from build123d import *

# Parameters (mm, degrees)
BOSS_EXTRUDE1_DEPTH             = 50
SKETCH2_W                       = 109.146932236
SKETCH2_H                       = 60.735636093
CUT_EXTRUDE1_DEPTH              = 88.05
F_20_0_161_DIAMETER_HOLE1_D     = 4.0894
F_20_0_161_DIAMETER_HOLE1_DEPTH = 87.05
SKETCH7_W                       = 11
SKETCH7_H                       = 4
BOSS_EXTRUDE2_DEPTH             = 20
FILLET1_R                       = 2
SKETCH8_R                       = 5.5
BOSS_EXTRUDE3_DEPTH             = 8
BOSS_EXTRUDE3_DEPTH_BACK        = 12
FILLET2_R                       = 5


with BuildPart() as part:
    # Sketch1 → Boss-Extrude1 (new body)
    with BuildSketch(Plane.XY):
        with BuildLine():
            Line((-86.473709878, 10), (-83.956551263, 10))
            ThreePointArc((-83.956551263, 10), (-84.55, 0), (-83.956551263, -10))
            Line((-83.956551263, -10), (-86.473709878, -10))
            ThreePointArc((-86.473709878, -10), (-87.05, 0), (-86.473709878, 10))
        make_face()
    extrude(amount=BOSS_EXTRUDE1_DEPTH)

    # Sketch2 → Cut-Extrude1 (cut, through all)
    with BuildSketch(Plane(origin=(0, 0, 0), x_dir=(0, 0, -1), z_dir=(1, 0, 0))):
        with Locations((-34.220207601, -2.682367057)):
            Rectangle(SKETCH2_W, SKETCH2_H)
        Polygon((0, 10), (0, -10), (-5, -10), (-50, -2.5), (-50, 2.5), (-5, 10), align=None, mode=Mode.SUBTRACT)
    extrude(amount=-CUT_EXTRUDE1_DEPTH, mode=Mode.SUBTRACT)

    # #20 (0.161) Diameter Hole1
    with Locations(Plane(origin=(0, 0, 0), x_dir=(0, 0, -1), z_dir=(1, 0, 0))):
        with Locations((-46, 0), (-5, 6), (-5, -6), (-17.5, 0)):
            Hole(F_20_0_161_DIAMETER_HOLE1_D / 2, depth=F_20_0_161_DIAMETER_HOLE1_DEPTH)

    # Sketch7 → Boss-Extrude2 (add)
    with BuildSketch(Plane(origin=(-80, 0, -87.99983), x_dir=(0, 0, -1), z_dir=(1, 0, 0))):
        with Locations((-120.49983, 0)):
            Rectangle(SKETCH7_W, SKETCH7_H)
    extrude(amount=-BOSS_EXTRUDE2_DEPTH)

    # Fillet1
    fillet1_edges = [part.edges().sort_by_distance(p)[0] for p in [
        (-87.027021666, -2, 32.5),
        (-87.05, 0, 27),
        (-87.027021666, 2, 32.5),
        (-87.05, 0, 38),
    ]]
    fillet(fillet1_edges, radius=FILLET1_R)

    # Sketch8 → Boss-Extrude3 (add, two sides)
    with BuildSketch(Plane.XZ.offset(2)) as boss_extrude3_sk:
        with Locations((-94.5, 32.5)):
            Circle(SKETCH8_R)
    extrude(amount=BOSS_EXTRUDE3_DEPTH)
    extrude(boss_extrude3_sk.sketch, amount=-BOSS_EXTRUDE3_DEPTH_BACK)

    # Fillet2
    fillet2_edges = [part.edges().sort_by_distance(p)[0] for p in [
        (-100, 0, 38),
        (-100, 0, 27),
    ]]
    fillet(fillet2_edges, radius=FILLET2_R)


solid = part.part
Design review of the part built by this model. Coordinates are the model's own, in mm. A direction names the side the tool comes from. Coordinates: 2 decimals unless noted, no trailing zeros. Write each loop counter-clockwise with the first axis right and the second up, starting at its lowest first coordinate (ties: lowest second). Pieces come first, ordered by that corner, then holes. Notation, with made-up numbers: (-26, -11) - (-16, -11) arc R24 cw to (-16, 22) - close; hole circle Ø2 at (10.25, 33.5). An arc over 180 degrees is marked (long way). Use one line per item in the form item = value.
Q1. The part is to be moulded in two halves that separate along Z. For faces 6 (the cylindrical face through (-99.995, 5.944, 32.742)), 7 (the cylindrical face through (-85.81, 0.61, 19.45)), 8 (the flat face through (-85.5, 6.2, 27.8)), 9 (the flat face through (-82, 0, 27)), say which applies: +Z half, -Z half, draft (parallel to the pull), parting line (faces both ways), or undercut.
Taken from the geometry:
face_6 = parting line
face_7 = undercut
face_8 = +Z half
face_9 = -Z half
Q2. Consider section C-C (z = 29). Write out the cut boundary in (x, y), plus the area to 3 significant figures.
Taken from the geometry:
outline = (-99, -2) - (-98.74, -2) - (-98.74, -10) - (-90.26, -10) - (-90.26, -2) - (-88.96, -2) arc R2 cw to (-86.96, -3.91) arc R87.05 ccw to (-86.84, -6) - (-84.34, -6) arc R84.55 cw to (-84.53, -2) - (-80, -2) - (-80, 2) - (-84.53, 2) arc R84.55 cw to (-84.34, 6) - (-86.84, 6) arc R87.05 ccw to (-86.96, 3.91) arc R2 cw to (-88.96, 2) - (-90.26, 2) - (-90.26, 10) - (-98.74, 10) - (-98.74, 2) - (-99, 2) - close
area = 233 mm^2
Q3. Machinability: for faces 1 (the flat face through (-86, 0, 50)), 2 (the cylindrical face through (-99.995, -5.944, 32.742)), 3 (the cylindrical face through (-87.56, -2.57, 32.39)), 4 (the flat face through (-85.5, -6.3, 27.2)), 5 (the flat face through (-92, 0, 27)), which of the approach directions +Z, -Z, +X, -X, +Y, -Y give a long, thin tool a straight path to every point of the face, cutting with its end or side? Answer none if there is none.
Taken from the geometry:
face_1 = +Z, +X, -X, +Y, -Y
face_2 = -Y
face_3 = +Z, -Z, -Y
face_4 = +Z, +X, -Y
face_5 = -Z, -X, +Y, -Y
Q4. For probe 1 along Z at (x, y) = (-85.1, 0); probe 2 along Y at (x, z) = (-85.2, 5); probe 3 along Y at (x, z) = (-85.65, 17.5), list the stretches that pass through material, from the lowest coordinate up.
Taken from the geometry:
probe_1 = 0 to 15.46, 19.54 to 43.96, 48.04 to 50
probe_2 = -10 to -8.04, -3.96 to 3.96, 8.04 to 10
probe_3 = -7.92 to -2.04, 2.04 to 7.92
Q5. Consider section A-A (y = 0). Write out the cut boundary in (x, z).
Taken from the geometry:
outline = (-100, 32) arc R5 ccw to (-95, 27) - (-89.05, 27) arc R2 cw to (-87.05, 25) - (-87.05, 19.54) - (-84.55, 19.54) - (-84.55, 27) - (-80, 27) - (-80, 38) - (-84.55, 38) - (-84.55, 43.96) - (-87.05, 43.96) - (-87.05, 40) arc R2 cw to (-89.05, 38) - (-95, 38) arc R5 ccw to (-100, 33) - close; (-87.05, 0) - (-84.55, 0) - (-84.55, 15.46) - (-87.05, 15.46) - close; (-87.05, 48.04) - (-84.55, 48.04) - (-84.55, 50) - (-87.05, 50) - close
Q6. Consider section D-D (y = -6). Write out the cut boundary in (x, z), plus the area to 3 significant figures.
Taken from the geometry:
outline = circle Ø11 at (-94.5, 32.5); (-86.84, 0) - (-84.34, 0) - (-84.34, 2.96) - (-86.84, 2.96) - close; (-86.84, 7.04) - (-84.34, 7.04) - (-84.34, 29) - (-86.84, 29) - close
area = 157 mm^2
Q7. Consider section B-B (z = 46). Write out the cut boundary in (x, y), plus the area to 3 significant figures.
Taken from the geometry:
outline = (-87.03, -2.04) arc R87.05 ccw to (-86.99, -3.17) - (-84.49, -3.17) arc R84.55 cw to (-84.53, -2.04) - close; (-87.03, 2.04) - (-84.53, 2.04) arc R84.55 cw to (-84.49, 3.17) - (-86.99, 3.17) arc R87.05 ccw to start
area = 5.61 mm^2
Q8. Insertion check: pin 1 Ø2.5 at (x, z) = (-82.5, 35) entering from -Y; pin 2 Ø4 at (y, z) = (4, 16.5) entering from +X; pin 3 Ø1.5 at (x, y) = (-91, 3.5) entering from +Z; pin 4 Ø4.5 at (x, y) = (-82.5, 0.5) entering from +Z. Each pin has a flat end and moves straight along its axis. Give the tip position at first contact, or say it passes through.
Taken from the geometry:
pin_1 = -2
pin_2 = -84.34
pin_3 = 37.26
pin_4 = 50
